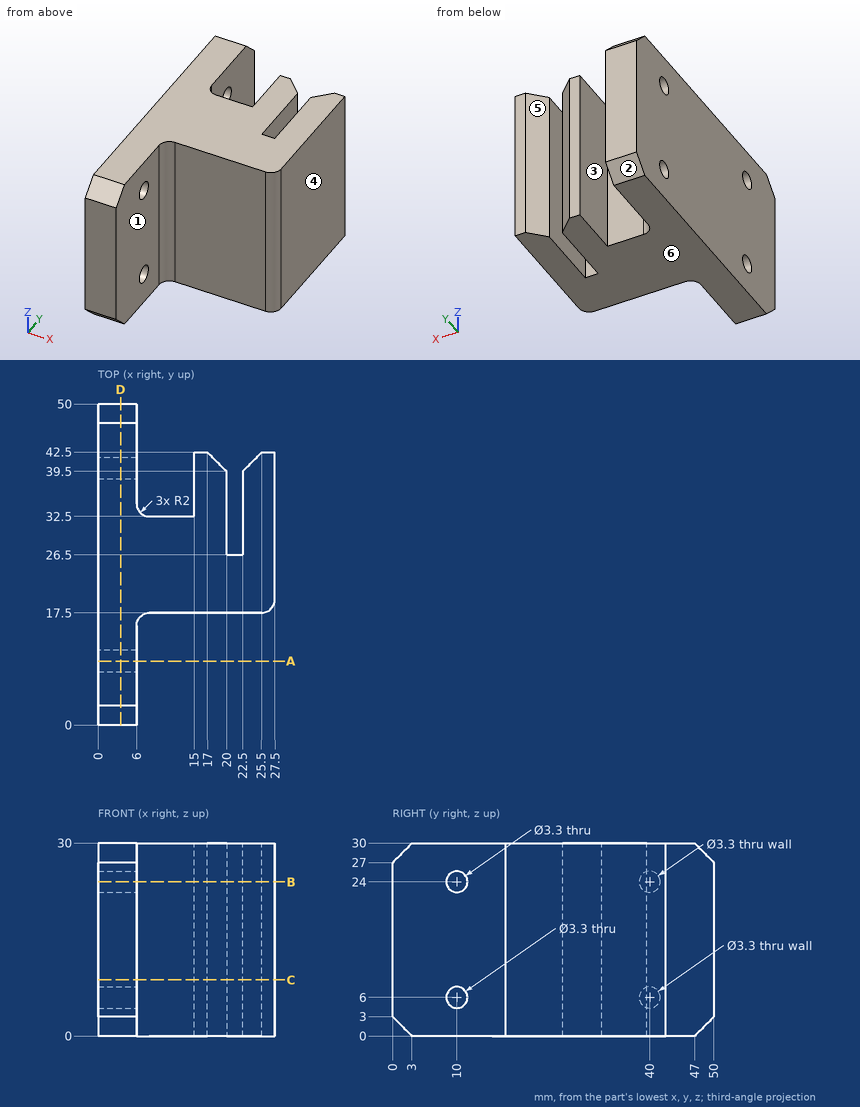
Geometry check sheet. Reference: drawing and pictorial views, mm from the part's lowest x, y, z. A direction names the side the tool comes from. Give positions to 0.01 mm unless a question says otherwise; leave off trailing zeros. Write each loop counter-clockwise with the first axis right and the second up, starting at its lowest first coordinate (ties: lowest second). Pieces come first, ordered by that corner, then holes. Notation, with made-up numbers: (62, 20.5) -> (112, 20.5) arc R21 ccw to (112, 35.5) -> close; hole circle Ø6 at (67, 27.5). An arc over 180 degrees is marked (long way). One line per item, written item: value. Start each with the question number.
Item 1: Section check B-B on z = 24. Record the cut outline in (x, y), then the cut area to 3 significant figures.
Item 2: Section check A-A on y = 10. Record the cut outline in (x, z).
Item 3: Section check C-C on z = 8.75. Record the cut outline in (x, y).
Item 4: Section check D-D on x = 3.5. Record the cut outline in (y, z).
Item 5: Gauge pin test, flat ends, axial feed: pin 1 (5 mm diameter, centred on x = 24, y = 43, fed in from -Z); pin 2 (2 mm diameter, centred on x = 20.5, z = 14, fed in from +Y); pin 3 (2 mm diameter, centred on x = 26.5, z = 16.5, fed in from +Y); pin 4 (12.5 mm diameter, centred on y = 4.5, z = 20, fed in from +X). Record the tip position at first contact, or that the pin passes through.
Item 6: Tool access check on the marked faces 1, 2 and 3. Record the directions out of +Z, -Z, +X, -X, +Y, -Y that give a thin tool (end or side, any length) a straight path to the whole face; none if there is none.
Item 7: Draft check along X on the marked faces 4, 5 and 6. Enter one of: +X half, -X half, draft (parallel to the pull), parting line (faces both ways), or undercut.
Item 8: Material ranges on probe 1 along X at (y, z) = (37.5, 27.5); probe 2 along Z at (x, y) = (2.5, 10); probe 3 along Y at (x, z) = (5.75, 4.5), recorded low to high. Write a range as from..to.
Results list:
1. outline: (0, 0) -> (6, 0) -> (6, 8.35) -> (0, 8.35) -> close; (0, 11.65) -> (6, 11.65) -> (6, 15.5) arc R2 cw to (8, 17.5) -> (25.5, 17.5) arc R2 ccw to (27.5, 19.5) -> (27.5, 42.5) -> (25.5, 42.5) -> (22.5, 39.5) -> (22.5, 26.5) -> (20, 26.5) -> (20, 39.5) -> (17, 42.5) -> (15, 42.5) -> (15, 32.5) -> (8, 32.5) arc R2 cw to (6, 34.5) -> (6, 38.35) -> (0, 38.35) -> close; (0, 41.65) -> (6, 41.65) -> (6, 50) -> (0, 50) -> close
1. area: 660 mm²
2. outline: (0, 0) -> (6, 0) -> (6, 4.35) -> (0, 4.35) -> close; (0, 7.65) -> (6, 7.65) -> (6, 22.35) -> (0, 22.35) -> close; (0, 25.65) -> (6, 25.65) -> (6, 30) -> (0, 30) -> close
3. outline: (0, 0) -> (6, 0) -> (6, 15.5) arc R2 cw to (8, 17.5) -> (25.5, 17.5) arc R2 ccw to (27.5, 19.5) -> (27.5, 42.5) -> (25.5, 42.5) -> (22.5, 39.5) -> (22.5, 26.5) -> (20, 26.5) -> (20, 39.5) -> (17, 42.5) -> (15, 42.5) -> (15, 32.5) -> (8, 32.5) arc R2 cw to (6, 34.5) -> (6, 50) -> (0, 50) -> close
4. outline: (0, 3) -> (3, 0) -> (47, 0) -> (50, 3) -> (50, 27) -> (47, 30) -> (3, 30) -> (0, 27) -> close; hole circle Ø3.3 at (10, 6); hole circle Ø3.3 at (10, 24); hole circle Ø3.3 at (40, 6); hole circle Ø3.3 at (40, 24)
5. pin 1: z = 0
5. pin 2: y = 40
5. pin 3: y = 42.5
5. pin 4: x = 6
6. face 1: +Z, -Z, +X, -Y
6. face 2: -Z, +X, -X, +Y
6. face 3: +Z, -Z, +Y
7. face 4: +X half
7. face 5: undercut
7. face 6: draft
8. probe 1: 0..6, 15..20, 22.5..27.5
8. probe 2: 0..4.35, 7.65..22.35, 25.65..30
8. probe 3: 0..9.31, 10.69..39.31, 40.69..50
